Geometry: final body of the model. Coordinates: model frame, mm. A direction names the side the tool comes from. Give positions to 0.01 mm unless a question says otherwise; leave off trailing zeros. Loops run counter-clockwise (first coordinate to the right, second up) from the corner with the lowest first, then second, coordinate; pieces in that order, holes last. Notation, with made-up numbers: (1.25, 60.25) -> (35.25, 60.25) arc R22 cw to (35.25, 68.25) -> close; hole circle Ø3 at (79, 23). An arc over 180 degrees is marked (long way). One line per question, with ' | ' between items. Start each with the question number.
Item 1: Section D-D on z = -10. Return loops of the section in (x, y), then the cut area to 3 significant figures.
Item 2: Material intervals for line 1 along Z through (x, y) = (7, -12); line 2 along X through (y, z) = (5.5, 5); line 3 along Z through (x, y) = (7, -2.75), sorted ascending. Write a range as [from, to].
Item 3: Section B-B on x = 7. Return loops of the section in (y, z).
Item 4: Set-up query: faces 1 (the flat face through (7, -11, -20)), 2 (the flat face through (9, -8.6, 7)). Return all of +Z, -Z, +X, -X, +Y, -Y with unobstructed straight access to the full face (end or side cutting, diameter ignored); none if empty.
Item 5: Pin query (flat end, axial travel): P1, Ø3, axis at x = 6.5, z = 0, coming from the +Y side; P2, Ø6.5, axis at x = 8, z = -10, coming from the +Y side; P3, Ø6, axis at y = -1.5, z = -13.5, coming from the -X side; P4, Ø1, axis at x = 10, y = 7.5, coming from the -Z side. Return the tip coordinate at first contact, or that it passes through.
Item 6: Section C-C on y = 4. Return loops of the section in (x, z).
Item 7: Mould query, pull axis X, two halves, no side actions, for faces 3 (the cylindrical face through (5.103, -11.845, 6.21)), 4 (the cylindrical face through (6.9, -5.17, -19.69)), 5 (the flat face through (14, -4, 5)). Classes: released by +X, released by -X, zero draft, split by the parting line, or undercut.
Item 8: Section A-A on z = 5. Return loops of the section in (x, y).
Autodesk Inventor part; units mm, degrees
ref_plane "Work Plane1" through (0, -4, -20) normal (0, -1, 0) x (1, 0, 0)
ref_plane "YZ Plane" through (0, 0, 0) normal (1, 0, 0) x (0, 1, 0)
ref_plane "XZ Plane" through (0, 0, 0) normal (0, 1, 0) x (-1, 0, 0)
sketch "Sketch1" plane through (0, 0, 0) normal (1, 0, 0) x (0, 1, 0)
  line L0 (15, 20) -> (-15, 20)
  line L1 (-15, 20) -> (-15, -20)
  line L2 (-15, -20) -> (15, -20)
  line L3 (15, -20) -> (15, 20)
  line L4 (15, 20) -> (-15, -20) construction
  line L5 (-15, 20) -> (15, -20) construction
  point P0 (0, 0)
  dimension "d0" = 30
  dimension "d1" = 40
extrude "Extrusion1" add sketch "Sketch1" along normal blind 14
sketch "Sketch2" plane through (14, 0, 0) normal (1, 0, 0) x (0, 0, -1)
  line L0 (-20, -15) -> (20, -15)
  line L1 (20, -15) -> (20, 15)
  line L2 (20, 15) -> (-20, 15)
  line L3 (-20, 15) -> (-20, -15)
  line L4 (-20, 15) -> (20, -5)
  point P0 (0, 0)
  dimension "d4" = 10
extrude "Extrusion2" cut sketch "Sketch2" against normal through all contours L2 L1 L4
fillet "Fillet1" radius 2 2 edges at (7, 15, 20) (7, -5, -20)
ref_plane "Work Plane1" through (0, -4, -20) normal (0, -1, 0) x (1, 0, 0)
sketch "Sketch3" plane through (0, -4, -20) normal (0, -1, 0) x (1, 0, 0)
  line L0 (0, 40) -> (14, 40)
  line L1 (0, 40) -> (14, 40)
  line L2 (14, 0) -> (0, 0)
  line L3 (0, 0) -> (14, 0)
  point P0 (0, 20)
  point P1 (7, 10)
  point P2 (7, 25)
  point P3 (7, 40)
  dimension "d9" = 15
  dimension "d10" = 10
hole "Hole1" at (7, -4, -10) at (7, -4, 5) direction (0, -1, 0) diameter 4.5 end through all counterbore diameter 8 counterbore depth 4.6
sketch "Sketch4" plane through (0, -4, -20) normal (0, -1, 0) x (1, 0, 0)
  circle A0 centre (7, 10) radius 4
  circle A1 centre (7, 10) radius 4
  circle A2 centre (7, 25) radius 4
  circle A3 centre (7, 25) radius 4
  point P0 (0, 20)
extrude "Extrusion3" cut sketch "Sketch4" against normal through all
properties part number "blokada_hiwin_3DPrint"
Result sheet:
1) outline: (0, -15) -> (4.75, -15) -> (4.75, -8.6) -> (3, -8.6) -> (3, 0) -> (0, 0) -> close; (9.25, -15) -> (14, -15) -> (14, 0) -> (11, 0) -> (11, -8.6) -> (9.25, -8.6) -> close | area: 112 mm²
2) line 1: z = [-20, -12.25], [-7.75, 2.75], [7.25, 20] | line 2: x = [0, 3], [11, 14] | line 3: z = [-15.5, -14], [-6, 1], [9, 20]
3) outline: (-15, -20) -> (-6.24, -20) arc R2 ccw to (-4.45, -18.89) -> (-2, -14) -> (-8.6, -14) -> (-8.6, -12.25) -> (-15, -12.25) -> close; (-15, -7.75) -> (-8.6, -7.75) -> (-8.6, -6) -> (2, -6) -> (5.5, 1) -> (-8.6, 1) -> (-8.6, 2.75) -> (-15, 2.75) -> close; (-15, 7.25) -> (-8.6, 7.25) -> (-8.6, 9) -> (9.5, 9) -> (13.55, 17.11) arc R2 ccw to (11.76, 20) -> (-15, 20) -> close
4) face 1: -Z, +X, -X, +Y, -Y | face 2: +Y
5) P1: stops at y = 5.62 | P2: stops at y = 1.19 | P3: stops at x = 0 | P4: stops at z = 6.94
6) outline: (0, -2) -> (14, -2) -> (14, 20) -> (0, 20) -> close; hole circle Ø8 at (7, 5)
7) face 3: undercut | face 4: zero draft | face 5: released by +X
8) outline: (0, -15) -> (4.75, -15) -> (4.75, -8.6) -> (3, -8.6) -> (3, 7.5) -> (0, 7.5) -> close; (9.25, -15) -> (14, -15) -> (14, 7.5) -> (11, 7.5) -> (11, -8.6) -> (9.25, -8.6) -> close
